Here's how the part is built. I have some questions about the finished solid (model axes, mm). Face numbers are marked on the shaded views. A direction names the side the tool comes from. Give positions to 0.01 mm unless a question says otherwise; leave off trailing zeros. Write each loop counter-clockwise with the first axis right and the second up, starting at its lowest first coordinate (ties: lowest second). Pieces come first, ordered by that corner, then holes. Notation, with made-up numbers: (30, -4.75) - (60, -4.75) arc R24 cw to (60, 6.25) - close; hole circle Ø10 at (32.5, 51.5). An arc over 180 degrees is marked (long way). Use one line per item in the form item = value. Start each with the question number.
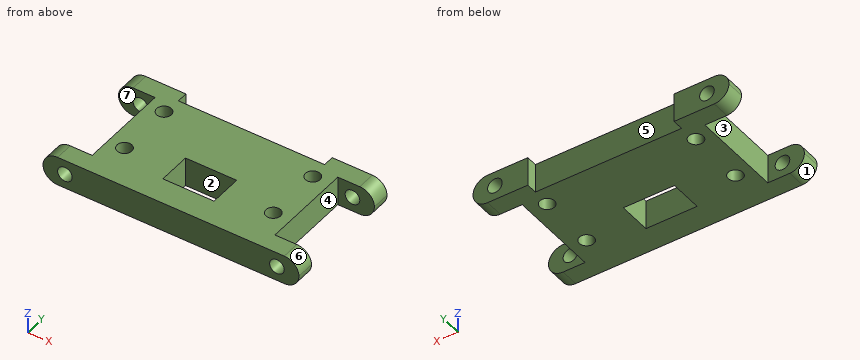
from build123d import *

# Parameters (mm, degrees)
SKETCH1_W           = 70
SKETCH1_H           = 35
BOSS_EXTRUDE1_DEPTH = 8
FILLET3_R           = 4
SKETCH7_R           = 2
CUT_EXTRUDE4_DEPTH  = 35
SKETCH8_R           = 2
SKETCH8_W           = 14
SKETCH8_H           = 9
CUT_EXTRUDE5_DEPTH  = 50.034709858
SKETCH10_W          = 40
SKETCH10_H          = 8
CUT_EXTRUDE6_DEPTH  = 3
SKETCH12_W          = 10
SKETCH12_H          = 25
CUT_EXTRUDE7_DEPTH  = 50.034709858


with BuildPart() as part:
    # Sketch1 → Boss-Extrude1 (new body)
    with BuildSketch(Plane.XY):
        with Locations((9.279257068, 1.987179487)):
            Rectangle(SKETCH1_W, SKETCH1_H)
    extrude(amount=BOSS_EXTRUDE1_DEPTH)

    # Fillet3
    fillet3_edges = [part.edges().sort_by_distance(p)[0] for p in [
        (44.279257068, 1.987179487, 0),
        (44.279257068, 1.987179487, 8),
        (-25.720742932, 1.987179487, 0),
        (-25.720742932, 1.987179487, 8),
    ]]
    fillet(fillet3_edges, radius=FILLET3_R - 0.0001)  # a hair under: the kernel refuses the full size

    # Sketch7 → Cut-Extrude4 (cut)
    with BuildSketch(Plane.XZ.offset(15.512820513)):
        with Locations((38.279257068, 4)):
            Circle(SKETCH7_R)
        with Locations((-19.720742932, 4)):
            Circle(SKETCH7_R)
    extrude(amount=-CUT_EXTRUDE4_DEPTH, mode=Mode.SUBTRACT)

    # Sketch8 → Cut-Extrude5 (cut, through all)
    with BuildSketch(Plane(origin=(0, 0, 0), x_dir=(-1, 0, 0), z_dir=(0, 0, -1))):
        with Locations((-29.494257068, -4.212820513)):
            Circle(SKETCH8_R)
        with Locations((-29.494257068, 11.487179487)):
            Circle(SKETCH8_R)
        with Locations((11.205742932, 11.487179487)):
            Circle(SKETCH8_R)
        with Locations((11.205742932, -4.212820513)):
            Circle(SKETCH8_R)
        with Locations((-9.144257068, -3.862820513)):
            Rectangle(SKETCH8_W, SKETCH8_H)
    extrude(amount=-CUT_EXTRUDE5_DEPTH, mode=Mode.SUBTRACT)

    # Sketch10 → Cut-Extrude6 (cut)
    with BuildSketch(Plane(origin=(0, 19.487179487, 0), x_dir=(1, 0, 0), z_dir=(0, 1, 0))):
        with Locations((9.279257068, -4)):
            Rectangle(SKETCH10_W, SKETCH10_H)
    extrude(amount=-CUT_EXTRUDE6_DEPTH, mode=Mode.SUBTRACT)

    # Sketch12 → Cut-Extrude7 (cut, through all)
    with BuildSketch(Plane(origin=(0, 0, 0), x_dir=(-1, 0, 0), z_dir=(0, 0, -1))):
        with Locations((20.720742932, 1.987179487)):
            Rectangle(SKETCH12_W, SKETCH12_H)
        with Locations((-39.279257068, 1.987179487)):
            Rectangle(SKETCH12_W, SKETCH12_H)
    extrude(amount=-CUT_EXTRUDE7_DEPTH, mode=Mode.SUBTRACT)


solid = part.part
1. For P1, Ø1, axis at y = 12, z = 3, coming from the +X side; P2, Ø4, axis at x = 16, z = 5.5, coming from the +Y side; P3, Ø0.9, axis at y = 17.5, z = 2.5, coming from the +X side, each with a flat end and sliding along its axis, tell me the tip position at first contact or that it passes through.
2. I want a section at C-C, the plane y = 10.5. List the corners of the cut face in (x, z) for me, then the cut area to 3 significant figures.
3. I want a section at D-D, the plane x = 17.5. List the corners of the cut face in (y, z) for me, then the cut area to 3 significant figures.
4. Please list where these lines run through material, in increasing order: line 1 (Y direction, x = -11, z = 1.5); line 2 (Y direction, x = 30.5, z = 2); line 3 (X direction, y = -2, z = 2).
5. I want a section at B-B, the plane y = 15.5. Give the number of separate pieces and of enclosed holes in the cut face, then the cut area to 3 significant figures.
6. I want a section at A-A, the plane x = 6. List the corners of the cut face in (y, z) for me, then the cut area to 3 significant figures.
7. We'd pull the mould along X, two halves only. Please class the marked faces 5, 6 and 7: pulls with the +X half, pulls with the -X half, needs draft (parallel to the pull), parting line crosses it, or undercut.
8. For the marked faces 1, 2, 3 and 4, which set-ups out of +Z, -Z, +X, -X, +Y, -Y let a thin tool reach every point of the face, with its end or its side?
Result sheet:
q1.P1 = 34.28
q1.P2 = 16.49
q1.P3 = 44.14
q2.outline = (-15.72, 0) - (-12.95, 0) - (-12.95, 8) - (-15.72, 8) - close; (-9.47, 0) - (27.75, 0) - (27.75, 8) - (-9.47, 8) - close; (31.23, 0) - (34.28, 0) - (34.28, 8) - (31.23, 8) - close
q2.area = 344 mm2
q3.outline = (-15.51, 0) - (16.49, 0) - (16.49, 8) - (-15.51, 8) - close
q3.area = 256 mm2
q4.line_1 = -15.51 to -6.2, -2.22 to 9.5, 13.48 to 19.49
q4.line_2 = -15.51 to -5.94, -2.48 to 9.76, 13.22 to 19.49
q4.line_3 = -15.72 to 2.14, 16.14 to 34.28
q5.separate_pieces = 1
q5.enclosed_holes = 2
q5.area = 521 mm2
q6.outline = (-15.51, 0) - (-8.36, 0) - (-8.36, 8) - (-15.51, 8) - close; (0.64, 0) - (16.49, 0) - (16.49, 8) - (0.64, 8) - close
q6.area = 184 mm2
q7.face_5 = undercut
q7.face_6 = pulls with the +X half
q7.face_7 = needs draft
q8.face_1 = -Z, -X, +Y, -Y
q8.face_2 = +Z, -Z
q8.face_3 = +Z, -Z, -X
q8.face_4 = +Z, -Z, +X
